Geometry: final body of the model. Coordinates: model frame, mm. A direction names the side the tool comes from. Round coordinates to 2 decimals unless told otherwise and drop trailing zeros. Order: outer loops, then holes, each group sorted by start corner. A loop starts at its lowest first (then second) coordinate and runs counter-clockwise, first axis right, second up. Notation, with made-up numbers: M 26.5,58 L 76.5,58 A30 ccw 76.5,92 Z; hole C 66.5,59.5 d8. An arc over 180 degrees is marked long. Return JSON: item names as keys, results as strings. Group by question number.
Q1. Contact query for flat-ended pins moving along their axis: pin 1 (5 mm diameter, centred on y = 24.5, z = 2.5, fed in from -X); pin 2 (1 mm diameter, centred on y = -50.8, z = 4.76, fed in from +X); pin 3 (1 mm diameter, centred on y = 15.5, z = 5, fed in from +X); pin 4 (1 mm diameter, centred on x = -16, z = 6.5, fed in from -Y). Output: stop coordinate, or through.
Q2. Cut plane A-A on z = 2.5. Output: boundary loops of the cut face in (x, y), and give its area (3 significant figures).
Q3. Access query for faces 1 (the face through (-31, 4.762, 5)), 2 (the face through (-31, -4.762, 5)), 3 (the face through (31, -4.762, 5)). Directions: +Z, -Z, +X, -X, +Y, -Y. A direction counts if a zero-diameter tool reaches every point of the face in a straight line with its end or side. Return the directions, or none.
Q4. Ray query, probe 1 along X at (y, z) = (50.8, 7); probe 2 along Y at (x, z) = (0, 5.75). Return the intervals inside material, ascending.
Q5. Cut plane B-B on y = 48. Output: boundary loops of the cut face in (x, z) (1 decimal), and give its area (3 significant figures).
```python
from build123d import *

# Parameters (mm, degrees)
F0_W     = 9.525
F0_H     = 52.3875
F0_W_2   = 52.3875
F0_H_2   = 9.525
F1_DEPTH = 9.525
F2_R     = 0.79375
F3_DEPTH = 9.525
F4_R     = 0.79375
F5_DEPTH = 9.525
F6_W     = 64.4
F6_H     = 21
F7_DEPTH = 11.15


# Not quite as in the source:
# - a length typed as a fraction of an inch, garbled in the dataset ("3 / 203.2 mm" for 3/8 in), is restored


with BuildPart() as f1:
    # F0 (on Top) → F1 (new body)
    with BuildSketch(Plane.XY):
        with Locations((0, 30.95625)):
            Rectangle(F0_W, F0_H)
        with Locations((30.95625, 0)):
            Rectangle(F0_W_2, F0_H_2)
        Rectangle(F0_W, F0_H_2)
        with Locations((0, -30.95625)):
            Rectangle(F0_W, F0_H)
        with Locations((-30.95625, 0)):
            Rectangle(F0_W_2, F0_H_2)
    extrude(amount=F1_DEPTH)

    # F2 (on face) → F3 (cut)
    with BuildSketch(Plane.XY.offset(9.525)):
        with Locations((0, 50.8)):
            Circle(F2_R)
        with Locations((50.8, 0)):
            Circle(F2_R)
        with Locations((-50.8, 0)):
            Circle(F2_R)
    extrude(amount=-F3_DEPTH, mode=Mode.SUBTRACT)

    # F4 (on face) → F5 (cut)
    with BuildSketch(Plane(origin=(-4.7625, 0, 0), x_dir=(0, -1, 0), z_dir=(-1, 0, 0))):
        with Locations((50.8, 4.7625)):
            Circle(F4_R)
    extrude(amount=-F5_DEPTH, mode=Mode.SUBTRACT)


with BuildPart() as f7:
    # F6 (on Top) → F7 (new body, symmetric)
    with BuildSketch(Plane.XY):
        with Locations((0, 0.8)):
            Rectangle(F6_W, F6_H)
    extrude(amount=F7_DEPTH, both=True)


solid = f1.part
```
Result sheet:
{
 "1": {"pin 1": "stops at x = -4.76", "pin 2": "passes through", "pin 3": "stops at x = 4.76", "pin 4": "stops at y = -4.76"},
 "2": {"outline": "M -57.15,-4.76 L -4.76,-4.76 L -4.76,-57.15 L 4.76,-57.15 L 4.76,-4.76 L 57.15,-4.76 L 57.15,4.76 L 4.76,4.76 L 4.76,57.15 L -4.76,57.15 L -4.76,4.76 L -57.15,4.76 Z; hole C -50.8,0 d1.59; hole C 0,50.8 d1.59; hole C 50.8,0 d1.59", "area": "2,080 mm²"},
 "3": {"face 1": "+Z, -Z, -X, +Y", "face 2": "+Z, -Z, -X, -Y", "face 3": "+Z, -Z, +X, -Y"},
 "4": {"probe 1": "x = -4.76 to -0.79, 0.79 to 4.76", "probe 2": "y = -57.15 to 50.01, 51.59 to 57.15"},
 "5": {"outline": "M -4.8,0 L 4.8,0 L 4.8,9.5 L -4.8,9.5 Z", "area": "90.7 mm²"}
}
